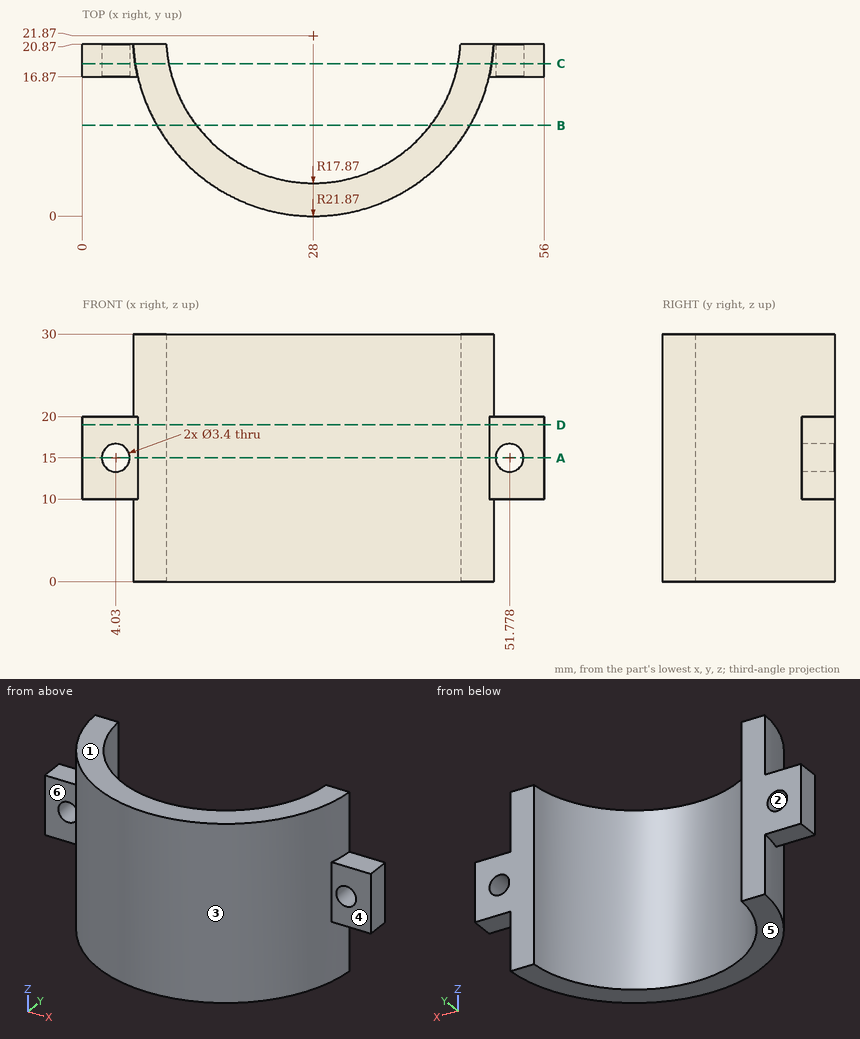
Can you work these out from the drawing? Everything is in mm from the part's minimum corner. A direction names the side the tool comes from. Give positions to 0.01 mm unless a question says otherwise; leave off trailing zeros. Loops run counter-clockwise (first coordinate to the right, second up) from the corner with the lowest first, then second, coordinate; pieces in that order, holes last. Notation, with made-up numbers: (62, 25) - (106, 25) arc R12 cw to (106, 48) - close; hole circle Ø1 at (-16.75, 12.5). An arc over 180 degrees is marked (long way). Answer as a JSON object with one key per item and string values.
Q1. Will these pins go through, and if not, where does the flat tip stop? P1, Ø4, axis at x = 32.5, z = 5, coming from the +Y side; P2, Ø1.5, axis at x = 16, z = 20.5, coming from the -Y side (1 decimal); P3, Ø4.5, axis at x = 2, y = 19.5, coming from the +Z side.
Geometry says:
{"P1": "y = 5.22", "P2": "y = 3.1", "P3": "z = 20"}
Q2. If I drill on L1, parallel to X at y = 19.7, z = 15; L2, parallel to X at y = 19, z = 15; L3, parallel to Y at x = 5, z = 11, over which ranges is the centre line in solid material (lowest first)?
Geometry says:
{"L1": "0 to 2.33, 5.73 to 10.26, 45.74 to 50.08, 53.48 to 56", "L2": "0 to 2.33, 5.73 to 10.36, 45.64 to 50.08, 53.48 to 56", "L3": "16.87 to 20.87"}
Q3. Imagine slicing it at A-A on z = 15. Write out the boundary of the cut face in (x, y).
Geometry says:
{"outline": "(0, 16.87) - (2.33, 16.87) - (2.33, 20.87) - (0, 20.87) - close; (5.73, 16.87) - (6.71, 16.87) arc R21.87 ccw to (49.29, 16.87) - (50.08, 16.87) - (50.08, 20.87) - (45.84, 20.87) arc R17.87 cw to (10.16, 20.87) - (5.73, 20.87) - close; (53.48, 16.87) - (56, 16.87) - (56, 20.87) - (53.48, 20.87) - close"}
Q4. Which directions (+Z, -Z, +X, -X, +Y, -Y) give clear straight access to the entire face, cutting with the end or side of a thin tool? Please do the marked faces 4, 5 and 6.
Geometry says:
{"face 4": "+Z, -Z, +X, -Y", "face 5": "-Z, +X, -X, +Y, -Y", "face 6": "+Z, -Z, -X, -Y"}
Q5. Imagine slicing it at B-B on y = 11. Write out the boundary of the cut face in (x, z), plus the area to 3 significant figures.
Geometry says:
{"outline": "(9.02, 0) - (13.82, 0) - (13.82, 30) - (9.02, 30) - close; (42.18, 0) - (46.98, 0) - (46.98, 30) - (42.18, 30) - close", "area": "288 mm²"}
Q6. Imagine slicing it at D-D on z = 19. Write out the boundary of the cut face in (x, y).
Geometry says:
{"outline": "(0, 16.87) - (6.71, 16.87) arc R21.87 ccw to (49.29, 16.87) - (56, 16.87) - (56, 20.87) - (45.84, 20.87) arc R17.87 cw to (10.16, 20.87) - (0, 20.87) - close"}
Q7. Imagine slicing it at C-C on y = 18.5. Write out the boundary of the cut face in (x, z), plus the area to 3 significant figures.
Geometry says:
{"outline": "(0, 10) - (6.39, 10) - (6.39, 0) - (10.45, 0) - (10.45, 30) - (6.39, 30) - (6.39, 20) - (0, 20) - close; (45.55, 0) - (49.61, 0) - (49.61, 10) - (56, 10) - (56, 20) - (49.61, 20) - (49.61, 30) - (45.55, 30) - close; hole circle Ø3.4 at (4.03, 15); hole circle Ø3.4 at (51.78, 15)", "area": "353 mm²"}
Q8. If we mould it in two halves opening along X, with no side actions, what happens to the marked faces 1, 2 and 3? For each: pulls with the +X half, pulls with the -X half, needs draft (parallel to the pull), parting line crosses it, or undercut.
Geometry says:
{"face 1": "needs draft", "face 2": "undercut", "face 3": "parting line crosses it"}
